Source: CAD feature listing. Evaluate the final solid. Frame: model axes, mm. Face numbers are marked on the shaded views. A direction names the side the tool comes from. Round coordinates to 2 decimals unless told otherwise and drop trailing zeros. Order: outer loops, then holes, each group sorted by start corner. A loop starts at its lowest first (then second) coordinate and runs counter-clockwise, first axis right, second up. Notation, with made-up numbers: (22.5, 0) -> (71.5, 0) arc R34 cw to (71.5, 39) -> close; hole circle Ø1 at (-5.5, -16). An arc over 180 degrees is marked (long way). Write item = value, one per line. Start each with the question number.
(1) Cut plane D-D on x = 3. Return the cut outline in (y, z).
(2) Cut plane C-C on z = 1. Return the cut outline in (x, y), then the cut area to 3 significant figures.
(3) Contact query for flat-ended pins moving along their axis: pin 1 Ø6.5 at (x, z) = (26, 6) entering from -Y; pin 2 Ø3 at (x, y) = (25.5, 7) entering from +Z; pin 3 Ø1.5 at (y, z) = (24.5, 8) entering from +X; pin 4 Ø5 at (x, z) = (26, 3.5) entering from -Y. Output: stop coordinate, or through.
(4) Reachability of the marked faces 5, 6, 7 and 8 from +Z, -Z, +X, -X, +Y, -Y: full face, straight path, thin tool, end or side. Return the list, or none.
(5) Cut plane B-B on y = 8. Return the cut outline in (x, z).
(6) Draft query along Y for the marked faces 1, 2, 3 and 4. Return one class per face: released by +Y, released by -Y, zero draft, split by the parting line, or undercut.
(7) Ray query, line 1 (X direction, y = 22, z = 10.5); line 2 (X direction, y = 7, z = 4.75); line 3 (Y direction, x = 16.5, z = 11.25). Return the intervals inside material, ascending.
(8) Cut plane A-A on x = 25. Return the cut outline in (y, z).
from build123d import *

# Parameters (mm, degrees)
SKETCH1_W           = 23.05
SKETCH1_H           = 26.67
BOSS_EXTRUDE1_DEPTH = 12
SKETCH2_W           = 12
SKETCH2_H           = 1.5
BOSS_EXTRUDE2_DEPTH = 4.75
FILLET1_R           = 0.5
SKETCH3_W           = 12
SKETCH3_H           = 1.5
BOSS_EXTRUDE3_DEPTH = 4.75
FILLET2_R           = 0.5
SKETCH4_W           = 6.2
SKETCH4_H           = 3.84
BOSS_EXTRUDE4_DEPTH = 6.03
SKETCH5_R           = 2.95
BOSS_EXTRUDE5_DEPTH = 9


with BuildPart() as part:
    # Sketch1 → Boss-Extrude1 (new body)
    with BuildSketch(Plane.XY):
        with Locations((11.525, 13.335)):
            Rectangle(SKETCH1_W, SKETCH1_H)
    extrude(amount=BOSS_EXTRUDE1_DEPTH)

    # Sketch2 → Boss-Extrude2 (add)
    with BuildSketch(Plane(origin=(23.05, 0, 0), x_dir=(0, 0, -1), z_dir=(1, 0, 0))):
        with Locations((-6, 21.05)):
            Rectangle(SKETCH2_W, SKETCH2_H)
    extrude(amount=BOSS_EXTRUDE2_DEPTH)

    # Fillet1
    fillet1_edges = [part.edges().sort_by_distance(p)[0] for p in [
        (27.8, 21.05, 12),
        (27.8, 21.05, 0),
    ]]
    fillet(fillet1_edges, radius=FILLET1_R)

    # Sketch3 → Boss-Extrude3 (add)
    with BuildSketch(Plane.ZY):
        with Locations((6, 21.05)):
            Rectangle(SKETCH3_W, SKETCH3_H)
    extrude(amount=BOSS_EXTRUDE3_DEPTH)

    # Fillet2
    fillet2_edges = [part.edges().sort_by_distance(p)[0] for p in [
        (-4.75, 21.05, 0),
        (-4.75, 21.05, 12),
    ]]
    fillet(fillet2_edges, radius=FILLET2_R)

    # Sketch4 → Boss-Extrude4 (add)
    with BuildSketch(Plane(origin=(23.05, 0, 0), x_dir=(0, 0, -1), z_dir=(1, 0, 0))):
        with Locations((-6, 6.97)):
            Rectangle(SKETCH4_W, SKETCH4_H)
    extrude(amount=BOSS_EXTRUDE4_DEPTH)

    # Sketch5 → Boss-Extrude5 (add)
    with BuildSketch(Plane(origin=(0, 26.67, 0), x_dir=(1, 0, 0), z_dir=(0, 1, 0))):
        with Locations(Location((16.395567503, -6.449737637, 0), (0, 0, 90))):
            Circle(SKETCH5_R)
    extrude(amount=BOSS_EXTRUDE5_DEPTH)


solid = part.part
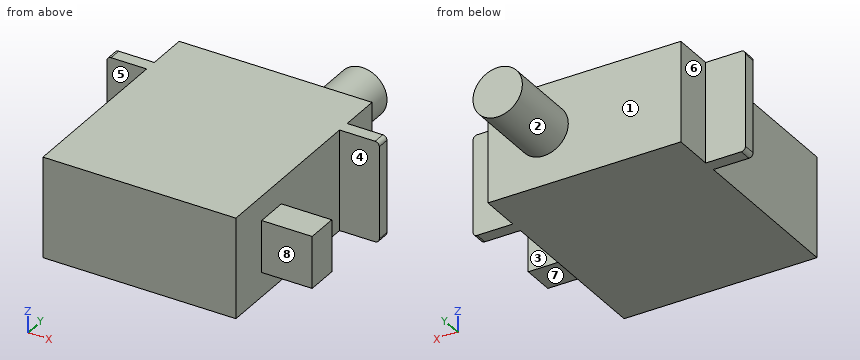
Evaluation:
q1.outline = (0, 0) -> (26.67, 0) -> (26.67, 12) -> (0, 12) -> close
q2.outline = (-4.75, 20.3) -> (0, 20.3) -> (0, 0) -> (23.05, 0) -> (23.05, 20.3) -> (27.8, 20.3) -> (27.8, 21.8) -> (23.05, 21.8) -> (23.05, 26.67) -> (0, 26.67) -> (0, 21.8) -> (-4.75, 21.8) -> close
q2.area = 629 mm^2
q3.pin_1 = 0
q3.pin_2 = 9.1
q3.pin_3 = 23.05
q3.pin_4 = 5.05
q4.face_5 = +Z, -Z, -X, -Y
q4.face_6 = +Z, -Z, -X, +Y
q4.face_7 = -Z, +X, -Y
q4.face_8 = +Z, -Z, +X, -Y
q5.outline = (0, 0) -> (23.05, 0) -> (23.05, 2.9) -> (29.08, 2.9) -> (29.08, 9.1) -> (23.05, 9.1) -> (23.05, 12) -> (0, 12) -> close
q6.face_1 = released by +Y
q6.face_2 = zero draft
q6.face_3 = undercut
q6.face_4 = undercut
q7.line_1 = 0 to 23.05
q7.line_2 = 0 to 29.08
q7.line_3 = 0 to 26.67
q8.outline = (5.05, 2.9) -> (8.89, 2.9) -> (8.89, 9.1) -> (5.05, 9.1) -> close; (20.3, 0) -> (21.8, 0) -> (21.8, 12) -> (20.3, 12) -> close
